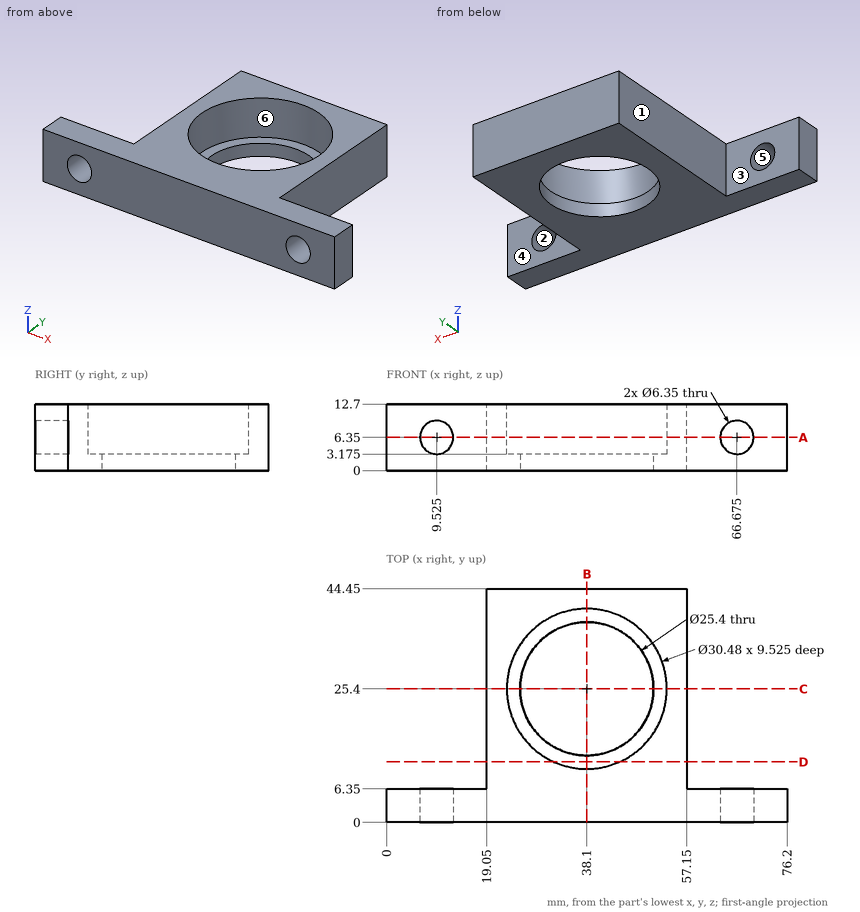
Geometry check sheet. Reference: drawing and pictorial views, mm from the part's lowest x, y, z. A direction names the side the tool comes from. Round coordinates to 2 decimals unless told otherwise and drop trailing zeros. Write each loop counter-clockwise with the first axis right and the second up, starting at its lowest first coordinate (ties: lowest second). Pieces come first, ordered by that corner, then holes.
Item 1: Material ranges on line 1 along Y through (x, z) = (38.1, 7); line 2 along Y through (x, z) = (9.5, 11.75); line 3 along X through (y, z) = (41, 2.5), recorded low to high.
Determined:
line 1: y = 0 to 10.16, 40.64 to 44.45
line 2: y = 0 to 6.35
line 3: x = 19.05 to 57.15
Item 2: Go/stop test with flat-tipped pins: pin 1 Ø24.5 at (x, y) = (38.1, 25.4) entering from -Z; pin 2 Ø5 at (x, y) = (37, 39.5) entering from +Z; pin 3 Ø6 at (y, z) = (16, 11.5) entering from -X; pin 4 Ø1 at (y, z) = (14.5, 5) entering from +X. Record where each tip stops, or that it passes through.
Determined:
pin 1: passes through
pin 2: stops at z = 12.7
pin 3: stops at x = 19.05
pin 4: stops at x = 57.15
Item 3: Access from +Z, -Z, +X, -X, +Y, -Y to the whole of each face (thin tool, end or side, straight path). Record for the marked faces 4, 5 and 6.
Determined:
face 4: +Z, -Z, +X, +Y
face 5: +Y, -Y
face 6: +Z
Item 4: Section check A-A (z = 6.35). Record the boundary of the cut face in (x, y), plus the area to 3 significant figures.
Determined:
outline: (0, 0) - (6.35, 0) - (6.35, 6.35) - (0, 6.35) - close; (12.7, 0) - (63.5, 0) - (63.5, 6.35) - (57.15, 6.35) - (57.15, 44.45) - (19.05, 44.45) - (19.05, 6.35) - (12.7, 6.35) - close; (69.85, 0) - (76.2, 0) - (76.2, 6.35) - (69.85, 6.35) - close; hole circle Ø30.48 at (38.1, 25.4)
area: 1,130 mm2
Item 5: Section check B-B (x = 38.1). Record the boundary of the cut face in (y, z) (3 decimals).
Determined:
outline: (0, 0) - (12.7, 0) - (12.7, 3.175) - (10.16, 3.175) - (10.16, 12.7) - (0, 12.7) - close; (38.1, 0) - (44.45, 0) - (44.45, 12.7) - (40.64, 12.7) - (40.64, 3.175) - (38.1, 3.175) - close
Item 6: Mould release check, pull along X, two halves, no side actions. Record for the marked faces 1, 2 and 3: +X half, -X half, draft (parallel to the pull), parting line (faces both ways), or undercut.
Determined:
face 1: -X half
face 2: undercut
face 3: draft
Item 7: Section check D-D (y = 11.5). Record the boundary of the cut face in (x, z) (3 decimals).
Determined:
outline: (19.05, 0) - (57.15, 0) - (57.15, 12.7) - (44.349, 12.7) - (44.349, 3.175) - (31.851, 3.175) - (31.851, 12.7) - (19.05, 12.7) - close
Item 8: Section check C-C (y = 25.4). Record the boundary of the cut face in (x, z) (3 decimals).
Determined:
outline: (19.05, 0) - (25.4, 0) - (25.4, 3.175) - (22.86, 3.175) - (22.86, 12.7) - (19.05, 12.7) - close; (50.8, 0) - (57.15, 0) - (57.15, 12.7) - (53.34, 12.7) - (53.34, 3.175) - (50.8, 3.175) - close
